```python
from build123d import *

# Parameters (mm, degrees)
F0_R     = 12.7
F0_R_2   = 9.525
F1_DEPTH = 4.7625
F2_W     = 38.1
F2_H     = 4.7625
F3_DEPTH = 4.7625
F4_W     = 4.7625
F4_H     = 88.9
F5_DEPTH = 4.7625
F7_DEPTH = 4.7625


with BuildPart() as f1:
    # F0 (on Top) → F1 (new body)
    with BuildSketch(Plane.XY):
        Circle(F0_R)
        Circle(F0_R_2, mode=Mode.SUBTRACT)
    extrude(amount=F1_DEPTH)

    # F2 (on face) → F3 (join)
    with BuildSketch(Plane.XY.offset(4.7625)):
        Rectangle(F2_W, F2_H)
    extrude(amount=-F3_DEPTH)

    # F4 (on face) → F5 (join)
    with BuildSketch(Plane.XY.offset(4.7625)):
        with Locations((0, -25.4)):
            Rectangle(F4_W, F4_H)
    extrude(amount=-F5_DEPTH)

    # F6 (on face) → F7 (join)
    with BuildSketch(Plane.XY.offset(4.7625)):
        Polygon((-2.38125, -66.675), (-2.38125, -53.975), (-11.90625, -53.975), (-11.90625, -57.15), (-8.73125, -57.15), (-8.73125, -60.325), (-5.55625, -60.325), (-5.55625, -63.5), (-11.90625, -63.5), (-11.90625, -66.675), align=None)
    extrude(amount=-F7_DEPTH)


solid = f1.part
```
The model under review builds one solid part; all positions refer to its coordinate system, in mm. A direction names the side the tool comes from. Round coordinates to 2 decimals unless told otherwise and drop trailing zeros. Order: outer loops, then holes, each group sorted by start corner. A loop starts at its lowest first (then second) coordinate and runs counter-clockwise, first axis right, second up.
(1) Take a section at B-B, the plane x = -6.5. State the section outline as (y, z) points (1 decimal), plus the area to 3 significant figures.
Working result:
outline: (-66.7, 0) - (-63.5, 0) - (-63.5, 4.8) - (-66.7, 4.8) - close; (-60.3, 0) - (-54, 0) - (-54, 4.8) - (-60.3, 4.8) - close; (-10.9, 0) - (-7, 0) - (-7, 4.8) - (-10.9, 4.8) - close; (-2.4, 0) - (2.4, 0) - (2.4, 4.8) - (-2.4, 4.8) - close; (7, 0) - (10.9, 0) - (10.9, 4.8) - (7, 4.8) - close
area: 106 mm2
(2) For P1, Ø2.5, axis at x = -6.5, z = 1.5, coming from the -Y side (3 decimals); P2, Ø2.5, axis at x = -7.5, z = 2.5, coming from the +Y side; P3, Ø2.5, axis at y = -65.5, z = 3, coming from the -X side, all flat-tipped, find the tip position at first contact; note any pin that passes through.
Working result:
P1: stops at y = -66.675
P2: stops at y = 11.06
P3: stops at x = -11.91
(3) Wall thickness on L1, parallel to Y at x = 8, z = 3; L2, parallel to Y at x = -10, z = 1.1 (3 decimals); L3, parallel to X at y = -6, z = 4.25: over which ranges is each line inside the solid? List them lowest first.
Working result:
L1: y = -9.86 to -5.17, -2.38 to 2.38, 5.17 to 9.86
L2: y = -66.675 to -63.5, -57.15 to -53.975, -7.829 to 7.829
L3: x = -11.19 to -7.4, -2.38 to 2.38, 7.4 to 11.19
(4) Take a section at D-D, the plane x = -14. State the section outline as (y, z) points, plus the area to 3 significant figures.
Working result:
outline: (-2.38, 0) - (2.38, 0) - (2.38, 4.76) - (-2.38, 4.76) - close
area: 22.7 mm2
(5) Tool access review of faces 5 (the face through (-9.055, -8.905, 2.348)), 6 (the face through (6, -2.381, 2)), 7 (the face through (2.381, -42, 2)), 8 (the face through (-2.381, 16, 2)): name each direction out of +Z, -Z, +X, -X, +Y, -Y from which nothing blocks a thin tool from reaching the whole face with its end or side.
Working result:
face 5: +Z, -Z, -X
face 6: +Z, -Z
face 7: +Z, -Z, +X, -Y
face 8: +Z, -Z, -X, +Y
(6) Take a section at C-C, the plane z = 0.95. Count the separate pieces of the cut face and the enclosed holes in it, plus the area to 3 significant figures.
Working result:
separate pieces: 1
enclosed holes: 4
area: 834 mm2
(7) Mouldability with a two-part tool opening along X and no side actions: class faces 1 (the face through (16, -2.381, 2)), 2 (the face through (-6.68, 6.79, 2.35)), 3 (the face through (19.05, 0, 2)), 4 (the face through (-6, -2.381, 2)) as released by +X, released by -X, zero draft, split by the parting line, or undercut.
Working result:
face 1: zero draft
face 2: undercut
face 3: released by +X
face 4: undercut
(8) Take a section at A-A, the plane y = -7.5. State the section outline as (x, z) points.
Working result:
outline: (-10.25, 0) - (-5.87, 0) - (-5.87, 4.76) - (-10.25, 4.76) - close; (-2.38, 0) - (2.38, 0) - (2.38, 4.76) - (-2.38, 4.76) - close; (5.87, 0) - (10.25, 0) - (10.25, 4.76) - (5.87, 4.76) - close
